Source: CAD feature listing. Evaluate the final solid. Frame: model axes, mm. Face numbers are marked on the shaded views. A direction names the side the tool comes from. Round coordinates to 2 decimals unless told otherwise and drop trailing zeros. Order: outer loops, then holes, each group sorted by start corner. A loop starts at its lowest first (then second) coordinate and runs counter-clockwise, first axis right, second up. Notation, with made-up numbers: (82.25, -10.75) -> (100.25, -10.75) arc R5 cw to (100.25, -6.75) -> close; hole circle Ø2 at (-16, 75.25). An arc over 180 degrees is marked (long way). Answer as CSV lines item,"result". Start each with the question number.
(1) Contact query for flat-ended pins moving along their axis: P1, Ø4, axis at y = 18.5, z = -2.5, coming from the -X side; P2, Ø6, axis at x = 73, z = -12.5, coming from the +Y side. Output: stop coordinate, or through.
(2) Section query B-B (y = 11). Output: boundary loops of the cut face in (x, z), plus the area to 3 significant figures.
(3) Set-up query: the marked faces 1 and 2. Return all of +Z, -Z, +X, -X, +Y, -Y with unobstructed straight access to the full face (end or side cutting, diameter ignored); none if empty.
(4) Section query A-A (x = 65). Output: boundary loops of the cut face in (y, z), plus the area to 3 significant figures.
(5) Line query: line 1 along Y through (x, z) = (108.9, -6); line 2 along Z through (x, y) = (65, 1.5); line 3 along X through (y, z) = (2.7, -6). Output: solid intervals per line, ascending. Write a range as from..to.
(6) Section query C-C (z = -6). Output: boundary loops of the cut face in (x, y).
(7) Section query D-D (z = -15). Output: boundary loops of the cut face in (x, y), plus the area to 3 significant figures.
```python
from build123d import *

# Parameters (mm, degrees)
SKETCH1_W           = 110
SKETCH1_H           = 20
BOSS_EXTRUDE1_DEPTH = 5
SKETCH2_W           = 5
SKETCH2_H           = 20
BOSS_EXTRUDE2_DEPTH = 52
SKETCH3_R           = 1.5
CUT_EXTRUDE1_DEPTH  = 6
FILLET1_R           = 8
SKETCH4_R           = 1.5
CUT_EXTRUDE2_DEPTH  = 6


with BuildPart() as part:
    # Sketch1 → Boss-Extrude1 (new body)
    with BuildSketch(Plane(origin=(0, 0, 0), x_dir=(1, 0, 0), z_dir=(0, 1, 0))):
        with Locations((55, 10)):
            Rectangle(SKETCH1_W, SKETCH1_H)
    extrude(amount=BOSS_EXTRUDE1_DEPTH)

    # Sketch2 → Boss-Extrude2 (add)
    with BuildSketch(Plane(origin=(0, 5, 0), x_dir=(1, 0, 0), z_dir=(0, 1, 0))):
        with Locations((107.5, 10)):
            Rectangle(SKETCH2_W, SKETCH2_H)
    extrude(amount=BOSS_EXTRUDE2_DEPTH)

    # Sketch3 → Cut-Extrude1 (cut, through all)
    with BuildSketch(Plane(origin=(0, 5, 0), x_dir=(1, 0, 0), z_dir=(0, 1, 0))):
        with Locations((6, 6)):
            Circle(SKETCH3_R)
        with Locations((65, 6)):
            Circle(SKETCH3_R)
    extrude(amount=-CUT_EXTRUDE1_DEPTH, mode=Mode.SUBTRACT)

    # Fillet1
    fillet1_edges = [part.edges().sort_by_distance(p)[0] for p in [
        (0, 2.5, 0),
        (0, 2.5, -20),
    ]]
    fillet(fillet1_edges, radius=FILLET1_R)

    # Sketch4 → Cut-Extrude2 (cut, through all)
    with BuildSketch(Plane.ZY.offset(-105)):
        with Locations((-6, 11)):
            Circle(SKETCH4_R)
        with Locations((-6, 51)):
            Circle(SKETCH4_R)
    extrude(amount=-CUT_EXTRUDE2_DEPTH, mode=Mode.SUBTRACT)


solid = part.part
```
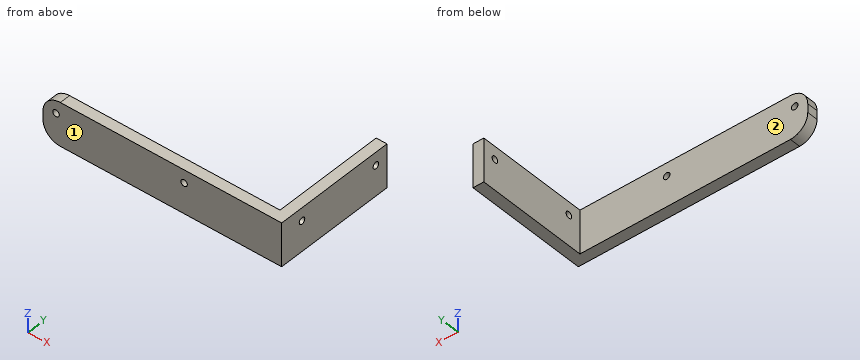
Answer block:
1,P1,"x = 105"
1,P2,"y = 5"
2,outline,"(105, -20) -> (110, -20) -> (110, -7.5) -> (105, -7.5) -> close; (105, -4.5) -> (110, -4.5) -> (110, 0) -> (105, 0) -> close"
2,area,"85.0 mm2"
3,face 1,"+Z, -Z, +X, -X, -Y"
3,face 2,"+Z, -Z, -X, +Y"
4,outline,"(0, -20) -> (5, -20) -> (5, -7.5) -> (0, -7.5) -> close; (0, -4.5) -> (5, -4.5) -> (5, 0) -> (0, 0) -> close"
4,area,"85.0 mm2"
5,line 1,"0..9.5, 12.5..49.5, 52.5..57"
5,line 2,"-20..-7.5, -4.5..0"
5,line 3,"0.25..4.5, 7.5..63.5, 66.5..110"
6,outline,"(0.25, 0) -> (4.5, 0) -> (4.5, 5) -> (0.25, 5) -> close; (7.5, 0) -> (63.5, 0) -> (63.5, 5) -> (7.5, 5) -> close; (66.5, 0) -> (110, 0) -> (110, 9.5) -> (105, 9.5) -> (105, 5) -> (66.5, 5) -> close; (105, 12.5) -> (110, 12.5) -> (110, 49.5) -> (105, 49.5) -> close; (105, 52.5) -> (110, 52.5) -> (110, 57) -> (105, 57) -> close"
7,outline,"(0.58, 0) -> (110, 0) -> (110, 57) -> (105, 57) -> (105, 5) -> (0.58, 5) -> close"
7,area,"807 mm2"
